Can you work these out from the model? Positions are in its coordinate system, mm. Face numbers are marked on the shaded views. A direction names the side the tool comes from. Round coordinates to 2 decimals unless told otherwise and drop trailing zeros. Write each loop counter-clockwise with the first axis right and the second up, starting at its lowest first coordinate (ties: lowest second). Pieces come first, ordered by that corner, then holes. Notation, with made-up numbers: (-32, -14) -> (-4, -14) arc R31 cw to (-4, 16) -> close; hole circle Ø5 at (-39, 88.25). An arc over 180 degrees is marked (long way). Write item = value, one per line. Start each with the question number.
1) For the marked faces 1, 2 and 3, which set-ups out of +Z, -Z, +X, -X, +Y, -Y let a thin tool reach every point of the face, with its end or its side?
2) I'm going to push flat-ended pins straight in: pin 1 (4 mm diameter, centred on x = -8.5, z = 2, fed in from +Y); pin 2 (10 mm diameter, centred on x = -19.5, z = 15, fed in from -Y); pin 3 (3 mm diameter, centred on x = -31.5, z = 17, fed in from +Y); pin 4 (2 mm diameter, centred on x = -11, y = 45.5, fed in from +Z). Where does each tip first touch, or does it pass through?
3) Imagine slicing it at B-B, the plane y = 36. State how many separate pieces and enclosed holes the cut face has, then the cut area to 3 significant figures.
4) Thinking about a two-plate mould opening in X: for the marked faces 4, 5 and 6, which applies, +X half, -X half, draft (parallel to the pull), parting line (faces both ways), or undercut?
5) Imagine slicing it at A-A, the plane x = -15.24. Please give me the cut outline in (y, z).
6) If I drill on line 1 (X direction, y = 25, z = 10); line 2 (Y direction, x = -1, z = 14.5); line 3 (Y direction, x = -23, z = 19.5), over which ranges is the centre line in solid material (lowest first)?
from build123d import *
from build123d.topology import SkipClean

# Parameters (mm, degrees)
SKETCH1_R           = 2.253608868
SKETCH1_R_2         = 1.535947569
BOSS_EXTRUDE1_DEPTH = 2.54
BOSS_EXTRUDE2_START = 2.54
SKETCH2_R           = 2.54
BOSS_EXTRUDE2_DEPTH = 2.54
SKETCH3_W           = 35.56
SKETCH3_H           = 12.390840881
BOSS_EXTRUDE3_DEPTH = 2.54
SKETCH4_R           = 12.7
BOSS_EXTRUDE4_DEPTH = 25.4


with BuildPart() as part:
    # Sketch1 → Boss-Extrude1 (new body)
    with BuildSketch(Plane(origin=(0, 0, 0), x_dir=(0, 0, -1), z_dir=(1, 0, 0))):
        with BuildLine():
            ThreePointArc((1.592468268, 1.978798831), (0.844230706, 2.395594815), (0, 2.54))
            Line((0, 2.54), (0, 4.244163865))
            add(Edge.make_bspline(
                [(0, 4.244163865), (-12.597388044, 22.987058756), (-10.054393134, 47.171038997)],
                knots=[0.08126898, 0.08126898, 0.08126898, 1, 1, 1], degree=2))
            Line((-10.054393134, 47.171038997), (-22.445234015, 47.171038997))
            add(Edge.make_bspline(
                [(-2.172846137, -1.315423759), (-29.204965898, 12.296498459), (-22.445234015, 47.171038997)],
                knots=[0, 0, 0, 1, 1, 1], degree=2))
            ThreePointArc((-2.172846137, -1.315423759), (1.146442405, -2.266554613), (2.347146338, 0.970826488))
            add(Edge.make_bspline(
                [(2.347146338, 0.970826488), (1.964088335, 1.472757402), (1.592468268, 1.978798831)],
                knots=[0, 0, 0, 0.025251884, 0.025251884, 0.025251884], degree=2))
        make_face()
        with Locations((-14.766403047, 22.09885284)):
            Circle(SKETCH1_R, mode=Mode.SUBTRACT)
        with Locations((-10.054393134, 10.254408813)):
            Circle(SKETCH1_R_2, mode=Mode.SUBTRACT)
        with BuildLine():
            ThreePointArc((-18.431438628, 40.801963274), (-18.282648873, 41.161173519), (-17.923438628, 41.309963274))
            Line((-17.923438628, 41.309963274), (-15.274403047, 41.309963274))
            ThreePointArc((-15.274403047, 41.309963274), (-14.915192802, 41.161173519), (-14.766403047, 40.801963274))
            Line((-14.766403047, 40.801963274), (-14.766403047, 34.017963549))
            ThreePointArc((-14.766403047, 34.017963549), (-14.915192802, 33.658753304), (-15.274403047, 33.509963549))
            Line((-15.274403047, 33.509963549), (-17.923438628, 33.509963549))
            ThreePointArc((-17.923438628, 33.509963549), (-18.282648873, 33.658753304), (-18.431438628, 34.017963549))
            Line((-18.431438628, 34.017963549), (-18.431438628, 40.801963274))
        make_face(mode=Mode.SUBTRACT)
    extrude(amount=BOSS_EXTRUDE1_DEPTH)

    # Sketch2 → Boss-Extrude2 (add)
    with SkipClean():  # the faces are left unmerged after this step: merging them gives an invalid solid
        with BuildSketch(Plane.ZY.offset(BOSS_EXTRUDE2_START)):
            Circle(SKETCH2_R)
        extrude(amount=-BOSS_EXTRUDE2_DEPTH)


with BuildPart() as body_2:
    # Mirror2: mirrored copy
    add(part.part.mirror(Plane.ZY.offset(15.24)))


with BuildPart() as part_1:
    with SkipClean():  # the faces are left unmerged after this step: merging them gives an invalid solid
        add(part.part)

        add(body_2.part)  # Boss-Extrude3 merges body 2
        # Sketch3 → Boss-Extrude3 (add)
        with BuildSketch(Plane(origin=(0, 47.171038997, 0), x_dir=(1, 0, 0), z_dir=(0, 1, 0))):
            with Locations((-15.24, -16.249813575)):
                Rectangle(SKETCH3_W, SKETCH3_H)
        extrude(amount=-BOSS_EXTRUDE3_DEPTH)

    # Sketch4 → Boss-Extrude4 (add)
    with SkipClean():  # the faces are left unmerged after this step: merging them gives an invalid solid
        with BuildSketch(Plane(origin=(0, 47.171038997, 0), x_dir=(1, 0, 0), z_dir=(0, 1, 0))):
            with Locations(Location((-15.24, -16.249813574, 0), (0, 0, 29.197947033))):
                Circle(SKETCH4_R)
        extrude(amount=BOSS_EXTRUDE4_DEPTH)


solid = part_1.part
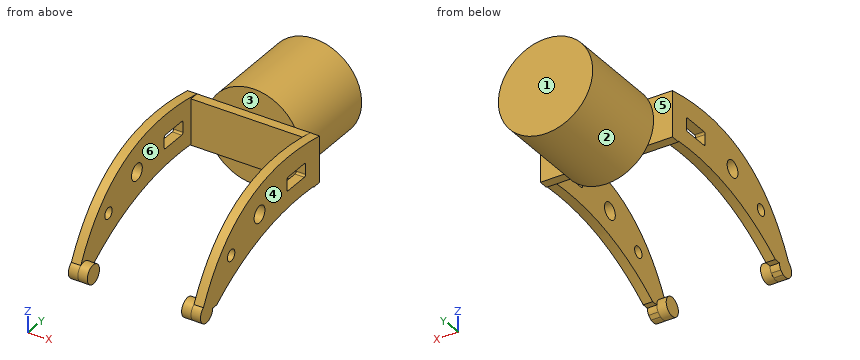
Reported:
q1.face_1 = +Z, -Z, +X, -X, +Y
q1.face_2 = +Y
q1.face_3 = +Z, +X, -X, -Y
q2.pin_1 = through
q2.pin_2 = 44.63
q2.pin_3 = 47.17
q2.pin_4 = 22.45
q3.separate_pieces = 4
q3.enclosed_holes = 0
q3.area = 49.2 mm²
q4.face_4 = +X half
q4.face_5 = draft
q4.face_6 = undercut
q5.outline = (44.63, 10.05) -> (47.17, 10.05) -> (47.17, 3.55) -> (72.57, 3.55) -> (72.57, 28.95) -> (47.17, 28.95) -> (47.17, 22.45) -> (44.63, 22.45) -> close
q6.line_1 = -33.02 to -30.48, 0 to 2.54
q6.line_2 = 44.63 to 47.17
q6.line_3 = 44.63 to 72.57
